```python
from build123d import *
from OCP.BRepFilletAPI import BRepFilletAPI_MakeFillet

# Parameters (mm, degrees)
BOSS_EXTRUDE2_DEPTH = 127
FILLET1_R1          = 1.5875
FILLET1_R2          = 1.4732
CUT_EXTRUDE1_DEPTH  = 50


with BuildPart() as part:
    # Sketch1 → Boss-Extrude2 (new body)
    with BuildSketch(Plane(origin=(0, 0, 0), x_dir=(1, 0, 0), z_dir=(0, 1, 0))):
        Polygon((-28.067579909, 0), (-28.067579909, -25.4), (-15.367579909, -25.4), (-15.367579909, -16.933333333), (-22.699928279, -21.166666582), (-22.699928279, -4.233333249), (-15.367579909, -8.466666667), (-15.367579909, 0), align=None)
    extrude(amount=BOSS_EXTRUDE2_DEPTH)

    # Fillet1: one fillet with a radius per group of edges: ONE call of the kernel's fillet builder (fillet() takes one radius for all edges)
    fillet1_edges_1 = [part.edges().sort_by_distance(p)[0] for p in [
        (-19.033754094, 127, 6.349999958),
        (-22.699928279, 127, 12.699999915),
        (-19.033754094, 127, 19.049999958),
        (-15.367579909, 127, 21.166666667),
        (-15.367579909, 127, 4.233333333),
        (-21.717579909, 127, 0),
        (-28.067579909, 63.5, 0),
        (-15.367579909, 63.5, 0),
        (-21.717579909, 0, 0),
        (-15.367579909, 0, 4.233333333),
        (-15.367579909, 63.5, 8.466666667),
        (-15.367579909, 63.5, 16.933333333),
        (-15.367579909, 0, 21.166666667),
        (-15.367579909, 63.5, 25.4),
        (-22.699928279, 0, 12.699999915),
        (-28.067579909, 127, 12.7),
        (-21.717579909, 127, 25.4),
        (-28.067579909, 63.5, 25.4),
        (-28.067579909, 0, 12.7),
        (-21.717579909, 0, 25.4),
        (-19.033754094, 0, 6.349999958),
        (-19.033754094, 0, 19.049999958),
    ]]
    fillet1_edges_2 = [part.edges().sort_by_distance(p)[0] for p in [
        (-22.699928279, 63.5, 4.233333249),
        (-22.699928279, 63.5, 21.166666582),
    ]]
    fillet1 = BRepFilletAPI_MakeFillet(part.part.solid().wrapped)
    for e in fillet1_edges_1:
        fillet1.Add(FILLET1_R1, e.wrapped)
    for e in fillet1_edges_2:
        fillet1.Add(FILLET1_R2, e.wrapped)
    add(Compound.cast(fillet1.Shape()), mode=Mode.REPLACE)

    # Sketch2 → Cut-Extrude1 (cut)
    with BuildSketch(Plane(origin=(0, 127, 0), x_dir=(1, 0, 0), z_dir=(0, 1, 0))):
        with BuildLine():
            Line((-23.422549559, -2.340780121), (-23.422549559, -4.963755825))
            ThreePointArc((-23.422549559, -4.963755825), (-27.722549476, -3.652267973), (-23.422549559, -2.340780121))
        make_face()
        with BuildLine():
            Line((-23.422549559, -23.059219761), (-23.422549559, -20.436244057))
            ThreePointArc((-23.422549559, -20.436244057), (-27.722549476, -21.747731909), (-23.422549559, -23.059219761))
        make_face()
    extrude(amount=-CUT_EXTRUDE1_DEPTH, mode=Mode.SUBTRACT)


solid = part.part
```
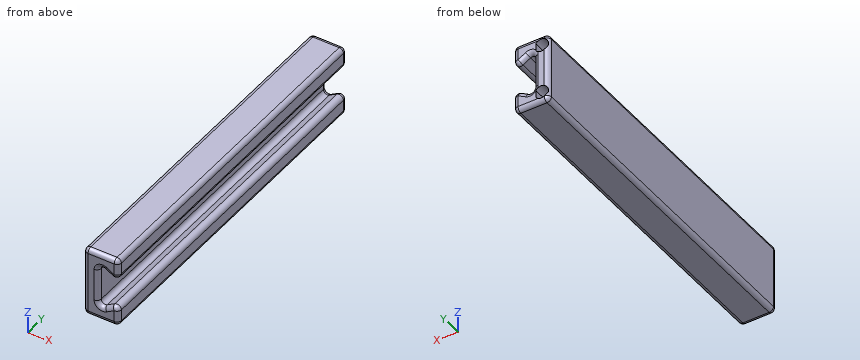
Check sheet for the modelled part. Datum: model origin and axes. Units: mm. Coordinates: 2 decimals unless noted, no trailing zeros. Write each loop counter-clockwise with the first axis right and the second up, starting at its lowest first coordinate (ties: lowest second). Pieces come first, ordered by that corner, then holes. Notation, with made-up numbers: (41.5, 42.25) - (69.5, 42.25) arc R12 ccw to (69.5, 47.25) - close; hole circle Ø5 at (48.5, 43). An arc over 180 degrees is marked (long way). One line per question, with ' | ' between items.
Item 1: Sectioned sample at A-A on y = 88. Give the number of separate pieces and of enclosed holes in the cut face, plus the area to 3 significant figures.
Determined:
separate pieces: 1 | enclosed holes: 2 | area: 194 mm2
Item 2: Thickness scan on line 1 (Z direction, x = -17, y = 110); line 2 (X direction, y = 109.5, z = 5.5); line 3 (X direction, y = 80, z = 17.75). Record the ranges inside material, lowest first. Write a range as [from, to].
Determined:
line 1: z = [0, 7.3], [18.1, 25.4] | line 2: x = [-28.07, -26.82], [-23.92, -21.95], [-20.51, -15.37] | line 3: x = [-28.07, -22.7]
Item 3: Gauge pin test, flat ends, axial feed: P1, Ø6, axis at x = -24.5, z = 14, coming from the -Y side; P2, Ø3.5, axis at y = 60, z = 11.5, coming from the +X side; P3, Ø6, axis at x = -20, z = 12, coming from the +Y side; P4, Ø1.3, axis at x = -25, z = 21.5, coming from the +Y side. Record the tip position at first contact, or that the pin passes through.
Determined:
P1: stops at y = 0 | P2: stops at x = -22.7 | P3: stops at y = 126.34 | P4: stops at y = 77
Item 4: Sectioned sample at C-C on z = 11.75. Record the boundary of the cut face in (x, y) (1 decimal).
Determined:
outline: (-28.1, 1.6) arc R1.6 ccw to (-26.5, 0) - (-24.3, 0) arc R1.6 ccw to (-22.7, 1.6) - (-22.7, 125.4) arc R1.6 ccw to (-24.3, 127) - (-26.5, 127) arc R1.6 ccw to (-28.1, 125.4) - close
Item 5: Sectioned sample at B-B on y = 72. Record the boundary of the cut face in (x, z) (1 decimal).
Determined:
outline: (-28.1, 1.6) arc R1.6 ccw to (-26.5, 0) - (-17, 0) arc R1.6 ccw to (-15.4, 1.6) - (-15.4, 5.7) arc R1.6 ccw to (-17.7, 7.1) - (-20.5, 5.5) arc R1.5 cw to (-22.7, 6.8) - (-22.7, 18.6) arc R1.5 cw to (-20.5, 19.9) - (-17.7, 18.3) arc R1.6 ccw to (-15.4, 19.7) - (-15.4, 23.8) arc R1.6 ccw to (-17, 25.4) - (-26.5, 25.4) arc R1.6 ccw to (-28.1, 23.8) - close
